```python
from build123d import *

# Parameters (mm, degrees)
F0_W     = 88.9
F0_H     = 33.655
F0_R     = 3.175
F1_DEPTH = 16.637
F3_DEPTH = 12.7
F5_DEPTH = 88.901


with BuildPart() as f1:
    # F0 (on Top) → F1 (new body)
    with BuildSketch(Plane.XY):
        Rectangle(F0_W, F0_H)
        with Locations((-38.1, 0)):
            Circle(F0_R, mode=Mode.SUBTRACT)
        with Locations((38.1, 0)):
            Circle(F0_R, mode=Mode.SUBTRACT)
    extrude(amount=-F1_DEPTH)

    # F2 (on face) → F3 (cut)
    with BuildSketch(Plane.XY):
        with BuildLine():
            Line((28.575, 5.2705), (-28.575, 5.2705))
            ThreePointArc((-28.575, 5.2705), (-31.9405, 1.905), (-28.575, -1.4605))
            Line((-28.575, -1.4605), (28.575, -1.4605))
            ThreePointArc((28.575, -1.4605), (31.9405, 1.905), (28.575, 5.2705))
        make_face()
    extrude(amount=-F3_DEPTH, mode=Mode.SUBTRACT)

    # F4 (on face) → F5 (cut, through all)
    with BuildSketch(Plane(origin=(-44.45, 0, 0), x_dir=(0, -1, 0), z_dir=(-1, 0, 0))):
        Polygon((16.8275, 0), (10.4775, 0), (16.8275, -6.35), align=None)
    extrude(amount=-F5_DEPTH, mode=Mode.SUBTRACT)


solid = f1.part
```
Part model, mm, in its own coordinate system. A direction names the side the tool comes from. Coordinates: 2 decimals unless noted, no trailing zeros. Order: outer loops, then holes, each group sorted by start corner. A loop starts at its lowest first (then second) coordinate and runs counter-clockwise, first axis right, second up. Notation, with made-up numbers: (55, -11) - (59, -11) arc R6 cw to (59, -3) - close; hole circle Ø6 at (16.5, 56). An arc over 180 degrees is marked (long way). Return JSON: item names as keys, results as strings. Group by question number.
Item 1: Pull direction Y, two halves, no side cores. Call faces 1 (the face through (-31.94, 1.98, -6.26)), 2 (the face through (-1, 6, 0)), 3 (the face through (0, -1.46, -6)), 4 (the face through (-1, -16.828, -11)): pulls with the +Y half, pulls with the -Y half, needs draft (parallel to the pull), parting line crosses it, or undercut.
Item 2: Which spindle directions (+Z, -Z, +X, -X, +Y, -Y) get a long thin tool onto all of the face, cutting with end or side? Do faces 5 (the face through (0, 5.27, -6)), 6 (the face through (-0.62, -13.61, -3.13)). Say none if no direction does.
Item 3: Pin check, flat tips, straight feed: pin 1 (10 mm diameter, centred on x = 38.1, y = 0, fed in from -Z); pin 2 (5 mm diameter, centred on x = -9, y = 2.5, fed in from +Z). Stop position of each tip, or through.
Item 4: Drill centre lines: probe 1 along Y at (x, z) = (-38.1, -11.5) (1 decimal); probe 2 along X at (y, z) = (1, -10.75); probe 3 along Y at (x, z) = (-15, -9.5). Where is each one in solid material? Low to high. Write a range as from..to.
Item 5: Cut at B-B (y = 0). List the corners of the cut face in (x, z) (3 decimals).
Item 6: Cut at A-A (z = -9). State how many separate pieces and enclosed holes the cut face has, plus the area to 3 significant figures.
Check values:
{
 "1": {"face 1": "undercut", "face 2": "needs draft", "face 3": "undercut", "face 4": "pulls with the -Y half"},
 "2": {"face 5": "+Z", "face 6": "+Z, +X, -X, -Y"},
 "3": {"pin 1": "stops at z = -16.64", "pin 2": "stops at z = -12.7"},
 "4": {"probe 1": "y = -16.8..-3.2, 3.2..16.8", "probe 2": "x = -44.45..-41.11, -35.09..-31.82, 31.82..35.09, 41.11..44.45", "probe 3": "y = -16.83..-1.46, 5.27..16.83"},
 "5": {"outline": "(-44.45, -16.637) - (-41.275, -16.637) - (-41.275, 0) - (-44.45, 0) - close; (-34.925, -16.637) - (34.925, -16.637) - (34.925, 0) - (31.349, 0) - (31.349, -12.7) - (-31.349, -12.7) - (-31.349, 0) - (-34.925, 0) - close; (41.275, -16.637) - (44.45, -16.637) - (44.45, 0) - (41.275, 0) - close"},
 "6": {"separate pieces": "1", "enclosed holes": "3", "area": "2,510 mm2"}
}
